```python
from build123d import *

# Parameters (mm, degrees)
SKETCH_1_R          = 1.65
EXTRUDE_1_DEPTH     = 3
SKETCH_2_W          = 12
SKETCH_2_H          = 3
EXTRUDE_2_DEPTH     = 22
CUT_EXTRUDE_2_DEPTH = 32
FILLET_1_R          = 2


with BuildPart() as part:
    # 草图1 → 凸台-拉伸1 (new body)
    with BuildSketch(Plane.XY):
        Polygon((-6, 16), (-13, 16), (-13, -3), (13, -3), (13, 16), (6, 16), (6, 19), (-6, 19), align=None)
        with Locations((-10, 0)):
            Circle(SKETCH_1_R, mode=Mode.SUBTRACT)
        with Locations((-5, 7.5)):
            Circle(SKETCH_1_R, mode=Mode.SUBTRACT)
        with Locations((10, 0)):
            Circle(SKETCH_1_R, mode=Mode.SUBTRACT)
        with Locations((5, 7.5)):
            Circle(SKETCH_1_R, mode=Mode.SUBTRACT)
    extrude(amount=EXTRUDE_1_DEPTH)

    # 草图2 → 凸台-拉伸2 (add)
    with BuildSketch(Plane(origin=(0, 0, 0), x_dir=(-1, 0, 0), z_dir=(0, 0, -1))):
        with Locations((0, 17.5)):
            Rectangle(SKETCH_2_W, SKETCH_2_H)
    extrude(amount=EXTRUDE_2_DEPTH)

    # 草图4 → 切除-拉伸2 (cut)
    with BuildSketch(Plane(origin=(0, 0, 0), x_dir=(1, 0, 0), z_dir=(0, 1, 0))):
        with BuildLine():
            Line((-1.65, 19), (-1.65, 16.5))
            ThreePointArc((-1.65, 16.5), (0, 14.85), (1.65, 16.5))
            Line((1.65, 16.5), (1.65, 19))
            ThreePointArc((1.65, 19), (0, 20.65), (-1.65, 19))
        make_face()
    extrude(amount=CUT_EXTRUDE_2_DEPTH, mode=Mode.SUBTRACT)

    # 圆角1
    fillet_1_edges = [part.edges().sort_by_distance(p)[0] for p in [
        (13, -3, 1.5),
        (-13, -3, 1.5),
        (-13, 16, 1.5),
        (13, 16, 1.5),
        (-6, 17.5, -22),
        (6, 17.5, -22),
    ]]
    fillet(fillet_1_edges, radius=FILLET_1_R)


solid = part.part
```
CAD build for the part. Positions are in the model's coordinates, mm. A direction names the side the tool comes from. Round coordinates to 2 decimals unless told otherwise and drop trailing zeros. Loops run counter-clockwise (first coordinate to the right, second up) from the corner with the lowest first, then second, coordinate; pieces in that order, holes last. Notation, with made-up numbers: M 74.25,16 L 112.25,16 A25 cw 112.25,41 Z; hole C 71,-19 d3. An arc over 180 degrees is marked long. Use a Markdown table: item, result. Add a question column.
(1) Which spindle directions (+Z, -Z, +X, -X, +Y, -Y) get a long thin tool onto all of the face, cutting with end or side? Do faces 4 (the face through (1.65, 17, -18)), 5 (the face through (12.4, 15.43, 1.52)), 6 (the face through (0, 16, -11)). Say none if no direction does.
(2) Cut at A-A (x = 0). Give the cut face in (y, z), and give its area (3 significant figures).
(3) Flat gauge pins, fed straight in: pin 1 (4 mm diameter, centred on x = -5, y = 7.5, fed in from -Z); pin 2 (1.5 mm diameter, centred on x = -8, z = 2, fed in from +Y); pin 3 (3 mm diameter, centred on x = -2.5, z = -4, fed in from -Y). Where does each tip first touch, or does it go through?
(4) Drill centre lines: line 1 (Y direction, x = -5, z = 1.8); line 2 (Y direction, x = -10, z = 2.2); line 3 (Z direction, x = -3.75, y = 0.5). Where is each one in solid material? Low to high.
(5) Cut at C-C (y = 7.5). Give the cut face in (x, z).
(6) Cut at B-B (z = -18.25). Give the cut face in (x, y).
(7) Cut at D-D (x = -5). Give the cut face in (y, z), and give its area (3 significant figures).
(8) Pull direction Y, two halves, no side cores. Call faces 1 (the face through (-6.65, 7.57, 1.48)), 2 (the face through (0.04, 17.48, -20.65)), 3 (the face through (0, -3, 1)): +Y half, -Y half, draft (parallel to the pull), parting line (faces both ways), or undercut.
Geometry says:
| question | item | result |
|---|---|---|
| 1 | face 4 | +Y, -Y |
| 1 | face 5 | +Z, -Z, +X, +Y |
| 1 | face 6 | -Z, +X, -X, -Y |
| 2 | outline | M -3,0 L 16,0 L 16,-14.85 L 19,-14.85 L 19,3 L -3,3 Z; M 16,-22 L 19,-22 L 19,-20.65 L 16,-20.65 Z |
| 2 | area | 115 mm² |
| 3 | pin 1 | stops at z = 0 |
| 3 | pin 2 | stops at y = 16 |
| 3 | pin 3 | stops at y = 16 |
| 4 | line 1 | y = -3 to 5.85, 9.15 to 19 |
| 4 | line 2 | y = -3 to -1.65, 1.65 to 16 |
| 4 | line 3 | z = 0 to 3 |
| 5 | outline | M -13,0 L -6.65,0 L -6.65,3 L -13,3 Z; M -3.35,0 L 3.35,0 L 3.35,3 L -3.35,3 Z; M 6.65,0 L 13,0 L 13,3 L 6.65,3 Z |
| 6 | outline | M -6,16 L -1.65,16 L -1.65,19 L -6,19 Z; M 1.65,16 L 6,16 L 6,19 L 1.65,19 Z |
| 7 | outline | M -3,0 L 5.85,0 L 5.85,3 L -3,3 Z; M 9.15,0 L 16,0 L 16,-21.73 L 19,-21.73 L 19,3 L 9.15,3 Z |
| 7 | area | 121 mm² |
| 8 | face 1 | undercut |
| 8 | face 2 | draft |
| 8 | face 3 | -Y half |
